The figure shows three views and two pictorial views of one solid part (mm, origin at its lowest corner). Answer the questions. A direction names the side the tool comes from. Coordinates: 2 decimals unless noted, no trailing zeros. Write each loop counter-clockwise with the first axis right and the second up, starting at its lowest first coordinate (ties: lowest second). Pieces come first, ordered by that corner, then holes. Notation, with made-up numbers: M 64.5,38 L 123.5,38 A6 cw 123.5,43 Z; hole C -13.5,26.5 d9. An arc over 180 degrees is marked long. Use CSV: the item, a comma, the result in double quotes.
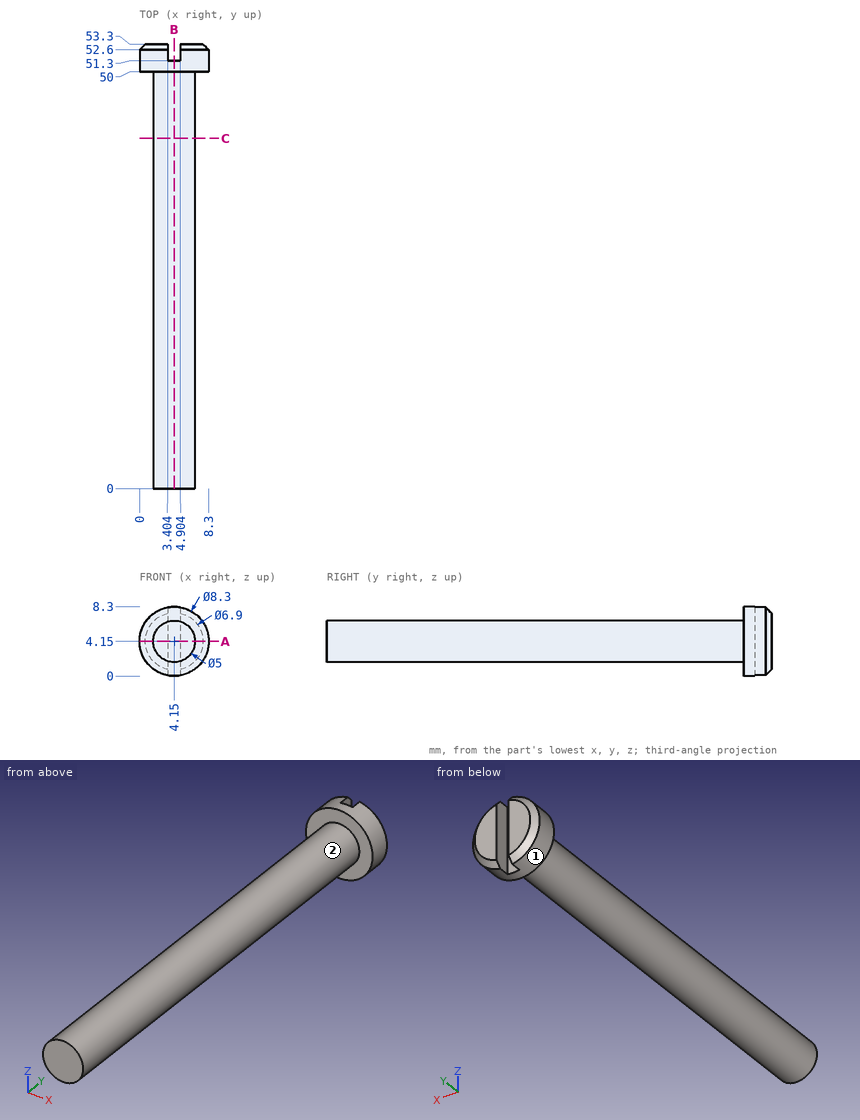
Item 1: The part is cut by section C-C (y = 42). Write down the section's boundary in (x, z).
Answer:
outline,"C 4.15,4.15 d5"
Item 2: A tool of negligible diameter and unlimited length cuts with its end or side. For the marked faces 1 and 2, from which of +Z, -Z, +X, -X, +Y, -Y can it reach the whole face along a straight path? Write none if from no direction.
Answer:
face 1,"+Y, -Y"
face 2,"-Y"
Item 3: The part is cut by section B-B (x = 4.15). Write down the section's boundary in (y, z).
Answer:
outline,"M 0,1.65 L 50,1.65 L 50,0 L 51.3,0 L 51.3,8.3 L 50,8.3 L 50,6.65 L 0,6.65 Z"
Item 4: Given pin 1 (3 mm diameter, centred on x = 6.5, y = 47.5, fed in from -Z); pin 2 (1.5 mm diameter, centred on x = 6, y = 42, fed in from +Z) (1 decimal); pin 3 (2 mm diameter, centred on x = 7, y = 6.5, fed in from +Z); pin 4 (4 mm diameter, centred on x = 3, z = 6, fed in from -Y), each flat-ended and moving along its own axis, determine where each tip first touches the part or whether it passes through.
Answer:
pin 1,"stops at z = 1.8"
pin 2,"stops at z = 6.4"
pin 3,"stops at z = 5.83"
pin 4,"stops at y = 0"
Item 5: Consider probe 1 along Y at (x, z) = (7, 5.75); probe 2 along Y at (x, z) = (3.5, 1.5); probe 3 along X at (y, z) = (22.5, 6). Determine where each line is inside the solid, lowest interval first.
Answer:
probe 1,"y = 50 to 53.3"
probe 2,"y = 50 to 51.3"
probe 3,"x = 2.47 to 5.83"
Item 6: The part is cut by section A-A (z = 4.15). Write down the section's boundary in (x, y), then the cut area to 3 significant figures.
Answer:
outline,"M 0,50 L 1.65,50 L 1.65,0 L 6.65,0 L 6.65,50 L 8.3,50 L 8.3,52.6 L 7.6,53.3 L 4.9,53.3 L 4.9,51.3 L 3.4,51.3 L 3.4,53.3 L 0.7,53.3 L 0,52.6 Z"
area,"274 mm2"
